from build123d import *

# Parameters (mm, degrees)
SKETCH2_R          = 3.15
SKETCH2_R_2        = 3.25
SKETCH2_R_3        = 3.1
MAINPLATE_DEPTH    = 6.5
PRESSFITNUTS_DEPTH = 5


with BuildPart() as part:
    # Sketch2 → MainPlate (new body)
    with BuildSketch(Plane(origin=(0, 0, 0), x_dir=(1, 0, 0), z_dir=(0, 1, 0))):
        with BuildLine():
            Line((24.899900609, -92.429929219), (0.2, -92.5))
            Line((0.2, -92.5), (-24.5, -92.5))
            ThreePointArc((-24.5, -92.5), (-27.871368271, -92.016678166), (-30.971160559, -90.605645997))
            Line((-30.971160559, -90.605645997), (-99.683475736, -46.605645997))
            ThreePointArc((-99.683475736, -46.605645997), (-104.578950448, -40.347025165), (-104.490786491, -32.401697323))
            Line((-104.490786491, -32.401697323), (-83.778471314, 24.598302677))
            ThreePointArc((-83.778471314, 24.598302677), (-80.773721892, 29.191692934), (-76.037940173, 31.966602781))
            Line((-76.037940173, 31.966602781), (-24.911380811, 47.741345462))
            ThreePointArc((-24.911380811, 47.741345462), (-22.845839779, 48.308813352), (-20.712315177, 48.5))
            Line((-20.712315177, 48.5), (0, 48.5))
            Line((0, 48.5), (20.712231832, 48.558758223))
            ThreePointArc((20.712231832, 48.558758223), (22.846290221, 48.373624884), (24.913432777, 47.812018957))
            Line((24.913432777, 47.812018957), (76.084537362, 32.182379345))
            ThreePointArc((76.084537362, 32.182379345), (80.828172093, 29.420915478), (83.845940292, 24.836067799))
            Line((83.845940292, 24.836067799), (104.719873926, -32.104944614))
            ThreePointArc((104.719873926, -32.104944614), (104.830577421, -40.049990373), (99.952877324, -46.322473865))
            Line((99.952877324, -46.322473865), (31.365661085, -90.517224974))
            ThreePointArc((31.365661085, -90.517224974), (28.26988419, -91.937045184), (24.899900609, -92.429929219))
        make_face()
        with Locations(Location((-72.5, 20.5, 0), (0, 0, 90))):
            Circle(SKETCH2_R, mode=Mode.SUBTRACT)
        with Locations(Location((-20.712315177, 36.5, 0), (0, 0, 90))):
            Circle(SKETCH2_R, mode=Mode.SUBTRACT)
        with Locations(Location((-93.212315177, -36.5, 0), (0, 0, 90))):
            Circle(SKETCH2_R, mode=Mode.SUBTRACT)
        with Locations(Location((-58.856157589, -58.5, 0), (0, 0, 90))):
            Circle(SKETCH2_R, mode=Mode.SUBTRACT)
        with Locations(Location((-24.5, -80.5, 0), (0, 0, 90))):
            Circle(SKETCH2_R, mode=Mode.SUBTRACT)
        with Locations(Location((-24.5, -36.5, 0), (0, 0, 90))):
            Circle(SKETCH2_R, mode=Mode.SUBTRACT)
        with Locations(Location((-72.5, -22.5, 0), (0, 0, 90))):
            Circle(SKETCH2_R, mode=Mode.SUBTRACT)
        with Locations(Location((24.74103568, -36.430154559, 0), (0, 0, 90))):
            Circle(SKETCH2_R, mode=Mode.SUBTRACT)
        with Locations(Location((24.865858124, -80.429977506, 0), (0, 0, 90))):
            Circle(SKETCH2_R, mode=Mode.SUBTRACT)
        with Locations(Location((59.159466244, -58.332601952, 0), (0, 0, 90))):
            Circle(SKETCH2_R, mode=Mode.SUBTRACT)
        with Locations(Location((93.453074364, -36.235226398, 0), (0, 0, 90))):
            Circle(SKETCH2_R, mode=Mode.SUBTRACT)
        with Locations(Location((72.701126299, -22.294040956, 0), (0, 0, 90))):
            Circle(SKETCH2_R, mode=Mode.SUBTRACT)
        with Locations(Location((72.579140729, 20.705786015, 0), (0, 0, 90))):
            Circle(SKETCH2_R, mode=Mode.SUBTRACT)
        with Locations(Location((20.746274317, 36.55880651, 0), (0, 0, 90))):
            Circle(SKETCH2_R, mode=Mode.SUBTRACT)
        with Locations(Location((0, -36.5, 0), (0, 0, 90))):
            Circle(SKETCH2_R_2, mode=Mode.SUBTRACT)
        with Locations(Location((0.182929062, -80.464988753, 0), (0, 0, 90))):
            Circle(SKETCH2_R_2, mode=Mode.SUBTRACT)
        with Locations(Location((0.103546099, -24.5, 0), (0, 0, 90))):
            Circle(SKETCH2_R_3, mode=Mode.SUBTRACT)
        with BuildLine():
            Line((3.105906565, 27.527701056), (3.193849827, 17.527701056))
            ThreePointArc((3.193849827, 17.527701056), (0.071672688, 14.350121804), (-3.105906565, 17.472298944))
            Line((-3.105906565, 17.472298944), (-3.193849827, 27.472298944))
            ThreePointArc((-3.193849827, 27.472298944), (-0.071672688, 30.649878196), (3.105906565, 27.527701056))
        make_face(mode=Mode.SUBTRACT)
    extrude(amount=MAINPLATE_DEPTH)

    # Sketch8 → PressFitNuts (cut)
    with BuildSketch(Plane(origin=(0, 6.5, 0), x_dir=(1, 0, 0), z_dir=(0, 1, 0))):
        Polygon((-4.835460238, -27.48990798), (0.223379197, -30.272258948), (5.162385534, -27.282350968), (5.042552437, -21.51009202), (-0.016286998, -18.727741052), (-4.955293335, -21.717649032), align=None)
        Polygon((-18.582159741, -36.5), (-21.54107987, -31.375), (-27.45892013, -31.375), (-30.417840259, -36.5), (-27.45892013, -41.625), (-21.54107987, -41.625), align=None)
        Polygon((-66.582159741, -22.5), (-69.54107987, -17.375), (-75.45892013, -17.375), (-78.417840259, -22.5), (-75.45892013, -27.625), (-69.54107987, -27.625), align=None)
        Polygon((-66.582159741, 20.5), (-69.54107987, 25.625), (-75.45892013, 25.625), (-78.417840259, 20.5), (-75.45892013, 15.375), (-69.54107987, 15.375), align=None)
        Polygon((-87.294474918, -36.5), (-90.253395048, -31.375), (-96.171235307, -31.375), (-99.130155436, -36.5), (-96.171235307, -41.625), (-90.253395048, -41.625), align=None)
        Polygon((-52.938317329, -58.5), (-55.897237459, -53.375), (-61.815077718, -53.375), (-64.773997848, -58.5), (-61.815077718, -63.625), (-55.897237459, -63.625), align=None)
        Polygon((-24.5, -74.582159741), (-29.625, -77.54107987), (-29.625, -83.45892013), (-24.5, -86.417840259), (-19.375, -83.45892013), (-19.375, -77.54107987), align=None)
        Polygon((-14.794474918, 36.5), (-17.753395048, 41.625), (-23.671235307, 41.625), (-26.630155436, 36.5), (-23.671235307, 31.375), (-17.753395048, 31.375), align=None)
        Polygon((17.753395048, 31.375), (14.794474918, 36.5), (17.753395048, 41.625), (23.671235307, 41.625), (26.630155436, 36.5), (23.671235307, 31.375), align=None)
        Polygon((19.375, -77.54107987), (24.5, -74.582159741), (29.625, -77.54107987), (29.625, -83.45892013), (24.5, -86.417840259), (19.375, -83.45892013), align=None)
        Polygon((55.897237459, -63.625), (52.938317329, -58.5), (55.897237459, -53.375), (61.815077718, -53.375), (64.773997848, -58.5), (61.815077718, -63.625), align=None)
        Polygon((90.253395048, -41.625), (87.294474918, -36.5), (90.253395048, -31.375), (96.171235307, -31.375), (99.130155436, -36.5), (96.171235307, -41.625), align=None)
        Polygon((69.54107987, 15.375), (66.582159741, 20.5), (69.54107987, 25.625), (75.45892013, 25.625), (78.417840259, 20.5), (75.45892013, 15.375), align=None)
        Polygon((69.54107987, -27.625), (66.582159741, -22.5), (69.54107987, -17.375), (75.45892013, -17.375), (78.417840259, -22.5), (75.45892013, -27.625), align=None)
        Polygon((21.54107987, -41.625), (18.582159741, -36.5), (21.54107987, -31.375), (27.45892013, -31.375), (30.417840259, -36.5), (27.45892013, -41.625), align=None)
    extrude(amount=-PRESSFITNUTS_DEPTH, mode=Mode.SUBTRACT)


solid = part.part
Work out the finished part from the listing and answer in its coordinate system (mm). A direction names the side the tool comes from. Coordinates: 2 decimals unless noted, no trailing zeros. Write each loop counter-clockwise with the first axis right and the second up, starting at its lowest first coordinate (ties: lowest second). Pieces come first, ordered by that corner, then holes. Notation, with made-up numbers: M 12.5,60.25 L 58.5,60.25 A26 ccw 58.5,81.25 Z; hole C 77.5,78.5 d1. An arc over 180 degrees is marked long. Answer as CSV lines item,"result". Start each with the question number.
Item 1: A tool of negligible diameter and unlimited length cuts with its end or side. For faces 4 (the face through (70, 1.5, -23)), 5 (the face through (1.245, 3.204, 33.498)), from which of +Z, -Z, +X, -X, +Y, -Y can it reach the whole face along a straight path? Write none if from no direction.
Item 2: Section A-A on x = -72.5 is taken. Write down the section's boundary in (y, z) (3 decimals).
Item 3: Consider L1, parallel to X at y = 0.5, z = 36.5; L2, parallel to Z at x = -24.5, y = 0.6; L3, parallel to Z at x = 73, y = 2 (3 decimals). Determine where each line is inside the solid, lowest interval first.
Item 4: Flat-ended cylindrical pins translate along their axes: P1, Ø3, axis at y = 4, z = -9, coming from the +X side; P2, Ø1, axis at y = 1, z = 58, coming from the -X side; P3, Ø2.5, axis at x = 73.5, y = 5, coming from the +Z side; P4, Ø4, axis at x = -72.5, z = -20.5, coming from the -Y side. Find the tip coordinate at first contact, or state that the pin passes through.
Item 5: Section B-B on y = 3 is taken. Give the number of separate pieces and of enclosed holes in the cut face, and give its area (3 significant figures).
Item 6: Determine the mould class of faces 1 (the face through (-104.542, 3.204, 40.454)), 2 (the face through (-12, 3, 92.5)), 3 (the face through (-88.795, 4.035, 39.098)) for opening direction X: released by +X, released by -X, zero draft, split by the parting line, or undercut.
Item 7: Section C-C on z = 0.5 is taken. Write down the section's boundary in (x, y), and give its area (3 significant figures).
Checks:
1,face 4,"+Y"
1,face 5,"+Y, -Y"
2,outline,"M 0,-33.058 L 6.5,-33.058 L 6.5,-25.625 L 1.5,-25.625 L 1.5,-23.65 L 0,-23.65 Z; M 0,-17.35 L 1.5,-17.35 L 1.5,-15.375 L 6.5,-15.375 L 6.5,17.375 L 1.5,17.375 L 1.5,19.35 L 0,19.35 Z; M 0,25.65 L 1.5,25.65 L 1.5,27.625 L 6.5,27.625 L 6.5,64.013 L 0,64.013 Z"
3,L1,"x = -105.21 to -96.36, -90.06 to -27.65, -21.35 to -3.25, 3.25 to 21.59, 27.89 to 90.31, 96.59 to 105.45"
3,L2,"z = -47.89 to 33.35, 39.65 to 77.35, 83.65 to 92.5"
3,L3,"z = -33.125 to -25.625, -15.375 to 17.375, 27.625 to 63.69"
4,P1,"stops at x = 90.2"
4,P2,"stops at x = -82.67"
4,P3,"stops at z = 64.17"
4,P4,"passes through"
5,separate pieces,"1"
5,enclosed holes,"18"
5,area,"20,900 mm²"
6,face 1,"released by -X"
6,face 2,"zero draft"
6,face 3,"undercut"
7,outline,"M -92.9,0 L 93.13,0 L 93.13,6.5 L -92.9,6.5 Z"
7,area,"1,210 mm²"
